Could you check a few things on this model? Use its own coordinates, in mm. Face numbers are marked on the shaded views. Give positions to 0.01 mm unless a question says otherwise; leave off trailing zeros. Order: outer loops, then holes, each group sorted by start corner. A loop starts at its lowest first (then second) coordinate and runs counter-clockwise, first axis right, second up. Notation, with made-up numbers: M -30,14 L -4,14 A10 cw -4,25 Z; hole C 77,85.25 d9. An arc over 180 degrees is marked long. Return JSON: item names as keys, results as strings. Group by question number.
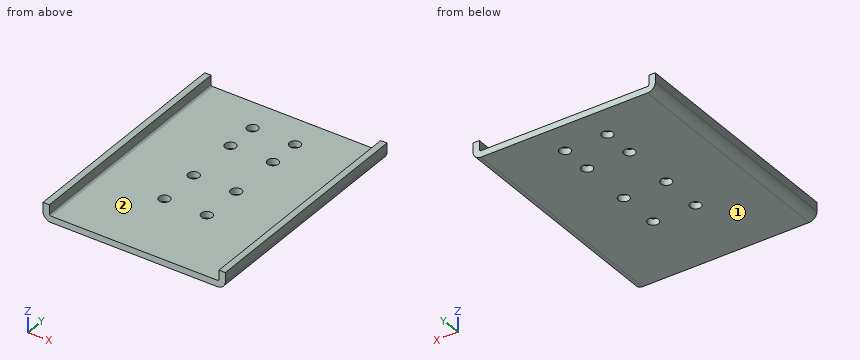
```python
from build123d import *

# Parameters (mm, degrees)
SKETCH1_W                      = 86
SKETCH1_H                      = 110
BASE_FLANGE1_DEPTH             = 3
SKETCH6_R                      = 2.58
CUT_EXTRUDE1_DEPTH             = 3
EDGE_FLANGE1_STRIP_W           = 13.4732
EDGE_FLANGE1_STRIP_H           = 3
EDGE_FLANGE1_STRIP_CUT_DEPTH   = 110
EDGE_FLANGE1_STRIP_2_W         = 13.4732
EDGE_FLANGE1_STRIP_2_H         = 3
EDGE_FLANGE1_STRIP_CUT_2_DEPTH = 110
EDGE_FLANGE1_DEPTH             = 110
EDGE_FLANGE1_BEND_DEPTH        = 110


# Sheet-metal steps are written as plain solids
with BuildPart() as part:
    # Sketch1 → Base-Flange1 (new body)
    with BuildSketch(Plane.XY):
        Rectangle(SKETCH1_W, SKETCH1_H)
    extrude(amount=-BASE_FLANGE1_DEPTH)

    # Sketch6 → Cut-Extrude1 (cut)
    with BuildSketch(Plane.XY):
        with Locations((-10, 40)):
            Circle(SKETCH6_R)
        with Locations((10, 40)):
            Circle(SKETCH6_R)
        with Locations((-10, 25)):
            Circle(SKETCH6_R)
        with Locations((10, 25)):
            Circle(SKETCH6_R)
        with Locations((10, 0)):
            Circle(SKETCH6_R)
        with Locations((-10, 0)):
            Circle(SKETCH6_R)
        with Locations((-10, -20)):
            Circle(SKETCH6_R)
        with Locations((10, -20)):
            Circle(SKETCH6_R)
    extrude(amount=-CUT_EXTRUDE1_DEPTH, mode=Mode.SUBTRACT)

    # Edge-Flange1 strip (across the edge) → Edge-Flange1 strip cut (cut)
    with BuildSketch(Plane(origin=(-43, 55, 0), x_dir=(1, 0, 0), z_dir=(0, -1, 0))):
        with Locations((-3, -1.5)):
            Rectangle(EDGE_FLANGE1_STRIP_W, EDGE_FLANGE1_STRIP_H)
    extrude(amount=EDGE_FLANGE1_STRIP_CUT_DEPTH, mode=Mode.SUBTRACT)

    # Edge-Flange1 strip 2 (across the edge) → Edge-Flange1 strip cut 2 (cut)
    with BuildSketch(Plane(origin=(43, -55, 0), x_dir=(-1, 0, 0), z_dir=(0, 1, 0))):
        with Locations((-3, -1.5)):
            Rectangle(EDGE_FLANGE1_STRIP_2_W, EDGE_FLANGE1_STRIP_2_H)
    extrude(amount=EDGE_FLANGE1_STRIP_CUT_2_DEPTH, mode=Mode.SUBTRACT)

    # Edge-Flange1 section (across the edge) → Edge-Flange1 (add)
    with BuildSketch(Plane(origin=(-43, 55, 0), x_dir=(1, 0, 0), z_dir=(0, -1, 0))):
        with BuildLine():
            Line((0, 0.7366), (0, 5))
            Line((0, 5), (3, 5))
            Line((3, 5), (3, 0.7366))
            ThreePointArc((3, 0.7366), (3.215745145, 0.215745145), (3.7366, 0))
            Line((3.7366, 0), (3.7366, -3))
            ThreePointArc((3.7366, -3), (1.094424801, -1.905575199), (0, 0.7366))
        make_face()
    extrude(amount=EDGE_FLANGE1_DEPTH)

    # Edge-Flange1 section 2 (across the edge) → Edge-Flange1 bend (add)
    with BuildSketch(Plane(origin=(43, -55, 0), x_dir=(-1, 0, 0), z_dir=(0, 1, 0))):
        with BuildLine():
            Line((0, 0.7366), (0, 5))
            Line((0, 5), (3, 5))
            Line((3, 5), (3, 0.7366))
            ThreePointArc((3, 0.7366), (3.215745145, 0.215745145), (3.7366, 0))
            Line((3.7366, 0), (3.7366, -3))
            ThreePointArc((3.7366, -3), (1.094424801, -1.905575199), (0, 0.7366))
        make_face()
    extrude(amount=EDGE_FLANGE1_BEND_DEPTH)


solid = part.part
```
1. Imagine slicing it at B-B, the plane x = -10. Please give me the cut outline in (y, z).
2. For pin 1 (6 mm diameter, centred on x = -10, y = 40, fed in from +Z); pin 2 (2 mm diameter, centred on y = -16, z = -0.5, fed in from -X), each with a flat end and sliding along its axis, tell me the tip position at first contact or that it passes through.
3. Imagine slicing it at C-C, the plane z = -1.5. Count the separate pieces of the cut face and the enclosed holes in it, plus the area to 3 significant figures.
4. I need wall thicknesses on L1, parallel to Y at x = -10, z = -1.85; L2, parallel to X at y = -44, z = 3; L3, parallel to X at y = 24, z = -0.5. Which ranges of each line are inside material? Lowest first, please. Write a range as from..to.
5. If we mould it in two halves opening along X, with no side actions, what happens to the marked faces 1 and 2? For each: pulls with the +X half, pulls with the -X half, needs draft (parallel to the pull), parting line crosses it, or undercut.
6. Imagine slicing it at A-A, the plane y = 0. Please give me the cut outline in (x, z), plus the area to 3 significant figures.
7. Imagine slicing it at D-D, the plane y = -46. Please give me the cut outline in (x, z), plus the area to 3 significant figures.
Values:
{
 "1": {"outline": "M -55,-3 L -22.58,-3 L -22.58,0 L -55,0 Z; M -17.42,-3 L -2.58,-3 L -2.58,0 L -17.42,0 Z; M 2.58,-3 L 22.42,-3 L 22.42,0 L 2.58,0 Z; M 27.58,-3 L 37.42,-3 L 37.42,0 L 27.58,0 Z; M 42.58,-3 L 55,-3 L 55,0 L 42.58,0 Z"},
 "2": {"pin 1": "stops at z = 0", "pin 2": "stops at x = -42.99"},
 "3": {"separate pieces": "1", "enclosed holes": "8", "area": "9,130 mm²"},
 "4": {"L1": "y = -55..-22.58, -17.42..-2.58, 2.58..22.42, 27.58..37.42, 42.58..55", "L2": "x = -43..-40, 40..43", "L3": "x = -42.79..-12.38, -7.62..7.62, 12.38..42.79"},
 "5": {"face 1": "needs draft", "face 2": "undercut"},
 "6": {"outline": "M -43,0.74 A3.74 ccw -39.26,-3 L -12.58,-3 L -12.58,0 L -39.26,0 A0.74 cw -40,0.74 L -40,5 L -43,5 Z; M -7.42,-3 L 7.42,-3 L 7.42,0 L -7.42,0 Z; M 12.58,-3 L 39.26,-3 A3.74 ccw 43,0.74 L 43,5 L 40,5 L 40,0.74 A0.74 cw 39.26,0 L 12.58,0 Z", "area": "251 mm²"},
 "7": {"outline": "M -43,0.74 A3.74 ccw -39.26,-3 L 39.26,-3 A3.74 ccw 43,0.74 L 43,5 L 40,5 L 40,0.74 A0.74 cw 39.26,0 L -39.26,0 A0.74 cw -40,0.74 L -40,5 L -43,5 Z", "area": "282 mm²"}
}
